from build123d import *

# Parameters (mm, degrees)
SKETCH1_R                    = 7.1374
BOSS_EXTRUDE1_DEPTH          = 23.5966
CHAMFER1_SIZE                = 0.254
CHAMFER2_SIZE                = 0.254
SKETCH2_R                    = 4.7625
CUT_EXTRUDE1_DEPTH           = 7.1755
SKETCH3_R                    = 6.35
CUT_EXTRUDE2_DEPTH           = 28.513757958
F_1_4_28_TAPPED_HOLE1_REACH  = 27.665
F_1_4_28_TAPPED_HOLE1_BORE_R = 2.7051


with BuildPart() as part:
    # Sketch1 → Boss-Extrude1 (new body)
    with BuildSketch(Plane(origin=(0, 0, 0), x_dir=(1, 0, 0), z_dir=(0, 1, 0))):
        with Locations(Location((0, 0, 0), (0, 0, 90))):
            Circle(SKETCH1_R)
    extrude(amount=BOSS_EXTRUDE1_DEPTH)

    # Chamfer1
    chamfer1_edges = [part.edges().sort_by_distance(p)[0] for p in [
        (0, 0, 7.1374),
    ]]
    chamfer(chamfer1_edges, length=CHAMFER1_SIZE)

    # Chamfer2
    chamfer2_edges = [part.edges().sort_by_distance(p)[0] for p in [
        (0, 23.5966, 7.1374),
    ]]
    chamfer(chamfer2_edges, length=CHAMFER2_SIZE)

    # Sketch2 → Cut-Extrude1 (cut, symmetric)
    with BuildSketch(Plane.XY):
        with Locations(Location((0, 11.7983, 0), (0, 0, 89.999999998))):
            Circle(SKETCH2_R)
    extrude(amount=CUT_EXTRUDE1_DEPTH, both=True, mode=Mode.SUBTRACT)

    # Sketch3 → Cut-Extrude2 (cut, through all)
    with BuildSketch(Plane.XY.offset(5.08)):
        with Locations((0, 11.7983)):
            Circle(SKETCH3_R)
    cut_extrude2 = extrude(amount=CUT_EXTRUDE2_DEPTH, mode=Mode.SUBTRACT)

    # Mirror1: Cut-Extrude2 across plane
    add(cut_extrude2.mirror(Plane.XY), mode=Mode.SUBTRACT)

    # 1/4-28 Tapped Hole1 bore → 1/4-28 Tapped Hole1 (cut, up to next)
    with BuildSketch(Plane(origin=(0, 0, 0), x_dir=(-1, 0, 0), z_dir=(0, -1, 0)), mode=Mode.PRIVATE) as f_1_4_28_tapped_hole1_sk1:
        Circle(F_1_4_28_TAPPED_HOLE1_BORE_R)
    f_1_4_28_tapped_hole1_tool1 = extrude(f_1_4_28_tapped_hole1_sk1.sketch, amount=-F_1_4_28_TAPPED_HOLE1_REACH, mode=Mode.PRIVATE) & part.part
    add(f_1_4_28_tapped_hole1_tool1.solids().sort_by_distance((0, 0, 0))[0], mode=Mode.SUBTRACT)


solid = part.part
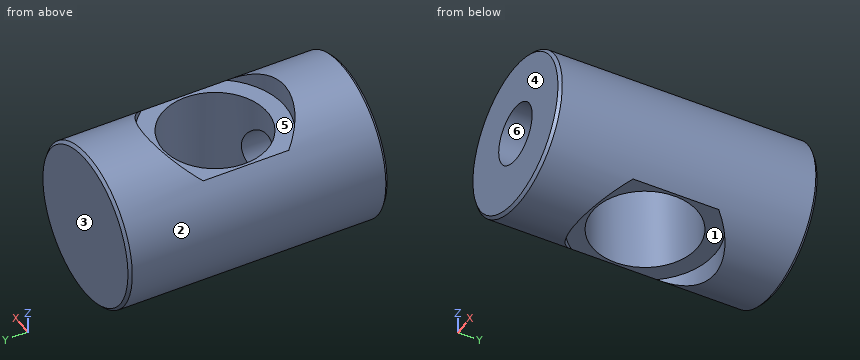
Input: part model. Units: mm. Frame: model coordinates. Face numbers are marked on the shaded views. A direction names the side the tool comes from. Give positions to 0.01 mm unless a question says otherwise; leave off trailing zeros. Loops run counter-clockwise (first coordinate to the right, second up) from the corner with the lowest first, then second, coordinate; pieces in that order, holes last. Notation, with made-up numbers: (71.25, 21) -> (78.25, 21) arc R21 cw to (78.25, 25) -> close; hole circle Ø9 at (-9, -26). An arc over 180 degrees is marked (long way). Answer as a JSON object with one key per item and string values. Group by question number.
Item 1: Cut plane A-A, the plane x = 0. Return the cut outline in (y, z), and give its area (3 significant figures).
Item 2: Pin query (flat end, axial travel): P1, Ø8, axis at x = -5, y = 3.5, coming from the -Z side; P2, Ø6, axis at y = 13.5, z = 3, coming from the -X side; P3, Ø1, axis at x = 0, y = 17, coming from the +Z side; P4, Ø1.5, axis at x = 5.5, y = 5, coming from the +Z side. Return the tip coordinate at first contact, or that it passes through.
Item 3: Cut plane D-D, the plane y = 8.75. Return the cut outline in (x, z).
Item 4: Pull-direction query (Y, two-part tool) for the marked faces 3, 4, 5 and 6; classes: released by +Y, released by -Y, zero draft, split by the parting line, or undercut.
Item 5: Cut plane B-B, the plane y = 12. Return the cut outline in (x, z).
Item 6: Line query: probe 1 along X at (y, z) = (2.75, 0); probe 2 along Z at (x, y) = (0, 5.75); probe 3 along X at (y, z) = (7.25, -1.5). Output: solid intervals per line, ascending.
Item 7: Reachability of the marked faces 1 and 2 from +Z, -Z, +X, -X, +Y, -Y: full face, straight path, thin tool, end or side. Return the list, or none.
Checks:
{
 "1": {"outline": "(0, -6.88) -> (0.25, -7.14) -> (5.45, -7.14) -> (5.45, -5.08) -> (7.04, -5.08) -> (7.04, -2.71) -> (0, -2.71) -> close; (0, 2.71) -> (7.04, 2.71) -> (7.04, 5.08) -> (5.45, 5.08) -> (5.45, 7.14) -> (0.25, 7.14) -> (0, 6.88) -> close; (16.56, -5.08) -> (18.15, -5.08) -> (18.15, -7.14) -> (23.34, -7.14) -> (23.6, -6.88) -> (23.6, 6.88) -> (23.34, 7.14) -> (18.15, 7.14) -> (18.15, 5.08) -> (16.56, 5.08) -> close", "area": "150 mm²"},
 "2": {"P1": "stops at z = -7.07", "P2": "stops at x = -7.14", "P3": "stops at z = 5.08", "P4": "stops at z = 5.33"},
 "3": {"outline": "(-5.01, -5.08) -> (-3.66, -5.08) -> (-3.66, 5.08) -> (-5.01, 5.08) arc R7.14 ccw to start; (3.66, -5.08) -> (5.01, -5.08) arc R7.14 ccw to (5.01, 5.08) -> (3.66, 5.08) -> close"},
 "4": {"face 3": "released by +Y", "face 4": "released by -Y", "face 5": "undercut", "face 6": "zero draft"},
 "5": {"outline": "(-5.01, -5.08) -> (-4.76, -5.08) -> (-4.76, 5.08) -> (-5.01, 5.08) arc R7.14 ccw to start; (4.76, -5.08) -> (5.01, -5.08) arc R7.14 ccw to (5.01, 5.08) -> (4.76, 5.08) -> close"},
 "6": {"probe 1": "x = -7.14 to -2.71, 2.71 to 7.14", "probe 2": "z = -5.08 to -2.71, 2.71 to 5.08", "probe 3": "x = -6.98 to -2.25, 2.25 to 6.98"},
 "7": {"face 1": "-Z", "face 2": "+Y, -Y"}
}
